Geometry check sheet. Reference: the model listing, model coordinates, mm. A direction names the side the tool comes from. Give positions to 0.01 mm unless a question says otherwise; leave off trailing zeros. Loops run counter-clockwise (first coordinate to the right, second up) from the corner with the lowest first, then second, coordinate; pieces in that order, holes last. Notation, with made-up numbers: (-26.75, 79.25) - (-2.75, 79.25) arc R8 ccw to (-2.75, 83.25) - close; hole circle Ø10 at (-32.75, 17.5). An arc over 180 degrees is marked (long way). Use a Markdown table: item, result. Add a question column.
1. Cross-section at A-A on y = 7. Enter the section's corners in (x, z).
2. Draft check along X on faces 1 (the cylindrical face through (-3.445, -0.624, -7.625)), 2 (the flat face through (0, -9.6, 2)), 3 (the flat face through (-4.912, -1, -11)), 4 (the flat face through (-14.12, -9.35, -1.02)). Enter one of: pulls with the +X half, pulls with the -X half, needs draft (parallel to the pull), parting line crosses it, or undercut.
3. Cross-section at D-D on z = -7. Enter the section's corners in (x, y), and give its area (3 significant figures).
4. Cross-section at C-C on y = -0.25. Enter the section's corners in (x, z) (1 decimal).
5. Depth check by flat-ended pin: P1, Ø5, axis at y = -6.5, z = 6.5, coming from the +X side; P2, Ø5, axis at x = -15, y = 5, coming from the -Z side; P3, Ø3.5, axis at y = 0.5, z = -11, coming from the -X side; P4, Ø6, axis at x = -3, z = -6.5, coming from the +Y side. Enter the tip coordinate at first touch or a pass-through.
6. Cross-section at B-B on x = -0.5. Enter the section's corners in (y, z) (3 decimals).
7. Set-up check for faces 5 (the flat face through (0, 4.22, 3)), 6 (the flat face through (4.912, -1, -11)), 7 (the flat face through (14.29, -9.35, -0.73)): record each of +Z, -Z, +X, -X, +Y, -Y from which the full face is reachable in a straight line by a thin tool's end or side.
8. Material ranges on L1, parallel to Z at x = -1, y = 2.75 (3 decimals); L2, parallel to Z at x = -8.5, y = -4.75; L3, parallel to Y at x = -2.5, z = -1.5, recorded low to high.
from build123d import *

# Parameters (mm, degrees)
BOSS_EXTRUDE1_DEPTH = 9.6
FILLET5_R           = 2
SKETCH7_W           = 10.46
SKETCH7_H           = 5.38
CUT_EXTRUDE6_DEPTH  = 34.879754173
SKETCH11_W          = 9.825
SKETCH11_H          = 9.825
CUT_EXTRUDE9_DEPTH  = 3.375
SKETCH12_R          = 1.5
CUT_EXTRUDE10_DEPTH = 9.825
CHAMFER1_SIZE       = 0.5


with BuildPart() as part:
    # Sketch1 → Boss-Extrude1 (new, symmetric)
    with BuildSketch(Plane(origin=(0, 0, 0), x_dir=(1, 0, 0), z_dir=(0, 1, 0))):
        Polygon((-14.297771125, -12.5), (14.297771125, -12.5), (22.216878365, -12.5), (7.783121635, 12.5), (-7.783121635, 12.5), (-22.216878365, -12.5), align=None)
    extrude(amount=BOSS_EXTRUDE1_DEPTH, both=True)

    # Fillet5
    fillet5_edges = [part.edges().sort_by_distance(p)[0] for p in [
        (-22.216878365, 0, 12.5),
        (-7.783121635, 0, -12.5),
        (7.783121635, 0, -12.5),
        (22.216878365, 0, 12.5),
    ]]
    fillet(fillet5_edges, radius=FILLET5_R)

    # Sketch7 → Cut-Extrude6 (cut, through all)
    with BuildSketch(Plane.XY.offset(12.5)):
        with Locations((0, 6.91)):
            Rectangle(SKETCH7_W, SKETCH7_H)
    extrude(amount=-CUT_EXTRUDE6_DEPTH, mode=Mode.SUBTRACT)

    # Sketch11 → Cut-Extrude9 (cut)
    with BuildSketch(Plane(origin=(0, 0, -12.5), x_dir=(-1, 0, 0), z_dir=(0, 0, -1))):
        with Locations((0, -0.6925)):
            Rectangle(SKETCH11_W, SKETCH11_H)
    extrude(amount=-CUT_EXTRUDE9_DEPTH, mode=Mode.SUBTRACT)

    # Sketch12 → Cut-Extrude10 (cut)
    with BuildSketch(Plane(origin=(0, 4.22, 0), x_dir=(1, 0, 0), z_dir=(0, 1, 0))):
        with Locations((3.4125, 9.125)):
            Circle(SKETCH12_R)
        with Locations((-3.4125, 9.125)):
            Circle(SKETCH12_R)
    extrude(amount=-CUT_EXTRUDE10_DEPTH, mode=Mode.SUBTRACT)

    # Chamfer1
    chamfer1_edges = [part.edges().sort_by_distance(p)[0] for p in [
        (-14.422649731, -9.6, -1),
        (0, -9.6, 12.5),
        (0, -9.6, -12.5),
        (14.422649731, -9.6, -1),
        (-20.484827557, -9.6, 11.5),
        (20.484827557, -9.6, 11.5),
        (7.628421097, -9.6, -12.232050808),
        (-7.628421097, -9.6, -12.232050808),
    ]]
    chamfer(chamfer1_edges, length=CHAMFER1_SIZE)


solid = part.part
Values found:
| question | item | result |
|---|---|---|
| 1 | outline | (-20.48, 9.5) - (-8.36, -11.5) arc R2 ccw to (-6.63, -12.5) - (-5.23, -12.5) - (-5.23, 12.5) - (-18.75, 12.5) arc R2 ccw to start; (5.23, -12.5) - (6.63, -12.5) arc R2 ccw to (8.36, -11.5) - (20.48, 9.5) arc R2 ccw to (18.75, 12.5) - (5.23, 12.5) - close |
| 2 | face 1 | undercut |
| 2 | face 2 | needs draft |
| 2 | face 3 | undercut |
| 2 | face 4 | pulls with the -X half |
| 3 | outline | (-10.96, -9.1) - (-10.38, -9.6) - (10.38, -9.6) - (10.96, -9.1) - (10.96, 9.6) - (5.23, 9.6) - (5.23, 4.22) - (-5.23, 4.22) - (-5.23, 9.6) - (-10.96, 9.6) - close |
| 3 | area | 364 mm2 |
| 4 | outline | (-20.5, 9.5) - (-8.4, -11.5) arc R2 ccw to (-6.6, -12.5) - (-4.9, -12.5) - (-4.9, -9.1) arc R1.5 cw to (-1.9, -9.1) - (1.9, -9.1) arc R1.5 cw to (4.9, -9.1) - (4.9, -12.5) - (6.6, -12.5) arc R2 ccw to (8.4, -11.5) - (20.5, 9.5) arc R2 ccw to (18.8, 12.5) - (-18.8, 12.5) arc R2 ccw to start |
| 5 | P1 | stops at x = 20.2 |
| 5 | P2 | stops at z = -4.33 |
| 5 | P3 | stops at x = -9.66 |
| 5 | P4 | stops at y = 9.6 |
| 6 | outline | (-9.6, -12) - (-9.1, -12.5) - (-5.605, -12.5) - (-5.605, -9.125) - (4.22, -9.125) - (4.22, 12.5) - (-9.1, 12.5) - (-9.6, 12) - close |
| 7 | face 5 | +Z, -Z, +Y |
| 7 | face 6 | -Z, +Y |
| 7 | face 7 | -Z, +X, -Y |
| 8 | L1 | z = -9.125 to 12.5 |
| 8 | L2 | z = -11.26 to 12.5 |
| 8 | L3 | y = -9.6 to 4.22 |
